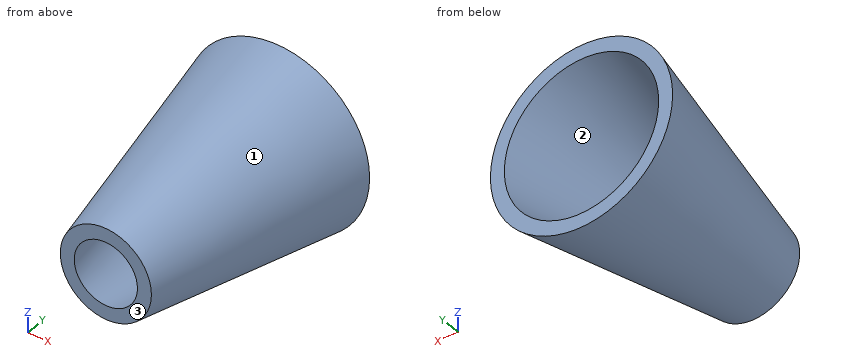
```python
from build123d import *

# Parameters (mm, degrees)
F0_R       = 10
F1_DEPTH   = 25
F1_FACE1_R = 10
F2_R       = 5
F4_T       = -1.5


with BuildPart() as f1:
    # F0 (on Front) → F1 (new body)
    with BuildSketch(Plane.XZ):
        Circle(F0_R)
    extrude(amount=F1_DEPTH)

    # F1_face1 (on face) → F3 section 0
    with BuildSketch(Plane(origin=(0, 0, 0), x_dir=(1, 0, 0), z_dir=(0, 1, 0))):
        Circle(F1_FACE1_R)
    # F2 (on face) → F3 section 1
    with BuildSketch(Plane.XZ.offset(25)):
        Circle(F2_R)
    loft(mode=Mode.INTERSECT)

    # F4
    f4_openings = [f1.faces().sort_by_distance(p)[0] for p in [
        (0, 0, 0),
        (0, -25, 0),
    ]]
    offset(amount=F4_T, openings=f4_openings, kind=Kind.INTERSECTION)


solid = f1.part
```
Here's how the part is built. I have some questions about the finished solid (model axes, mm). Face numbers are marked on the shaded views. Coordinates: 2 decimals unless noted, no trailing zeros. Write each loop counter-clockwise with the first axis right and the second up, starting at its lowest first coordinate (ties: lowest second). Pieces come first, ordered by that corner, then holes. Notation, with made-up numbers: (48, 7.25) -> (60, 7.25) arc R11 cw to (60, 28.25) -> close; hole circle Ø3 at (-38.5, 87.25). An arc over 180 degrees is marked (long way). Use a Markdown table: item, result. Add a question column.
(1) Please list where these lines run through material, in increasing order: line 1 (X direction, y = -10, z = 0.75); line 2 (X direction, y = -15, z = 0.5); line 3 (Z direction, x = 1.75, y = -4.75).
(2) I'm going to push flat-ended pins straight in: P1, Ø1, axis at x = 3, y = -17, coming from the -Z side; P2, Ø5, axis at x = 4, y = -16, coming from the +Z side; P3, Ø10, axis at x = -4.5, y = -22, coming from the +Z side. Where does each tip first touch, or does it pass through?
(3) If we section it at A-A, the plane x = 0: Write out the boundary of the cut face in (y, z).
(4) We'd pull the mould along Z, two halves only. Please class the marked faces 1, 2 and 3: +Z half, -Z half, draft (parallel to the pull), parting line (faces both ways), or undercut.
(5) If we section it at B-B, the plane y = -13.5: Write out the boundary of the cut face in (x, z).
Outcome:
| question | item | result |
|---|---|---|
| 1 | line 1 | x = -7.96 to -6.43, 6.43 to 7.96 |
| 1 | line 2 | x = -6.98 to -5.45, 5.45 to 6.98 |
| 1 | line 3 | z = -8.88 to -7.31, 7.31 to 8.88 |
| 2 | P1 | stops at z = -6.13 |
| 2 | P2 | stops at z = 6.81 |
| 2 | P3 | stops at z = 6.24 |
| 3 | outline | (-25, -5) -> (0, -10) -> (0, -8.47) -> (-25, -3.47) -> close; (-25, 3.47) -> (0, 8.47) -> (0, 10) -> (-25, 5) -> close |
| 4 | face 1 | parting line |
| 4 | face 2 | undercut |
| 4 | face 3 | draft |
| 5 | outline | circle Ø14.6 at (0, 0); hole circle Ø11.54 at (0, 0) |
